Can you work these out from the model? Positions are in its coordinate system, mm. A direction names the side the tool comes from. Round coordinates to 2 decimals unless told otherwise and drop trailing zeros. Write each loop counter-clockwise with the first axis right and the second up, starting at its lowest first coordinate (ties: lowest second). Pieces come first, ordered by that corner, then holes. Notation, with made-up numbers: M 73,32 L 90,32 A13 ccw 90,51 Z; hole C 29,-15.5 d1. An arc over 180 degrees is marked long. Answer in a Markdown table with one row per item. Add a question column.
(1) Suppose I cut it at B-B, the plane z = 16. Write out the boundary of the cut face in (x, y), then the cut area to 3 significant figures.
(2) For faces 5 (the face through (24.653, 28.694, 7.972)), 6 (the face through (28, 2, 0)), 7 (the face through (28, 17, 18)), 8 (the face through (-13, 36, 8)), which set-ups out of +Z, -Z, +X, -X, +Y, -Y let a thin tool reach every point of the face, with its end or its side?
(3) If we mould it in two halves opening along Y, with no side actions, what happens to faces 1 (the face through (32.77, 18.5, -13.25)), 2 (the face through (-27.4, 35.43, -7.97)), 3 (the face through (2.176, 36.842, -7.972)), 4 (the face through (21, 39, 8))? For each: released by +Y, released by -Y, zero draft, split by the parting line, or undercut.
(4) Suppose I cut it at C-C, the plane x = -7.5. Write out the boundary of the cut face in (y, z), then the cut area to 3 significant figures.
(5) Suppose I cut it at D-D, the plane z = 25. Write out the boundary of the cut face in (x, y), then the cut area to 3 significant figures.
(6) If I drill on probe 1 along Z at (x, y) = (11, 3.1); probe 2 along Z at (x, y) = (24, 18); probe 3 along Z at (x, y) = (9.5, 48), over which ranges is the centre line in solid material (lowest first)?
(7) Suppose I cut it at A-A, the plane y = 17. Write out the boundary of the cut face in (x, z), then the cut area to 3 significant figures.
(8) I'm going to push flat-ended pins straight in: pin 1 (14 mm diameter, centred on x = 12.5, y = 19.5, fed in from -Z); pin 2 (6 mm diameter, centred on x = 22, z = -18.5, fed in from -Y); pin 3 (6 mm diameter, centred on x = 4.5, z = 2, fed in from +Y); pin 4 (1.2 mm diameter, centred on y = 2.5, z = 5.5, fed in from +X). Where does each tip first touch, or does it pass through?
from build123d import *

# Parameters (mm, degrees)
SKETCH1_R           = 3.5
BOSS_EXTRUDE1_DEPTH = 4
BOSS_EXTRUDE2_DEPTH = 4
SKETCH6_R           = 5
BOSS_EXTRUDE3_DEPTH = 12


with BuildPart() as part:
    # Sketch1 → Boss-Extrude1 (new body)
    with BuildSketch(Plane(origin=(0, 0, 0), x_dir=(1, 0, 0), z_dir=(0, 1, 0))):
        Polygon((-28, 23), (-18, 33), (12, 33), (28, 17), (28, -17), (12, -33), (-18, -33), (-28, -23), align=None)
        with Locations((11, 25)):
            Circle(SKETCH1_R, mode=Mode.SUBTRACT)
        with Locations((11, -25)):
            Circle(SKETCH1_R, mode=Mode.SUBTRACT)
        with Locations((-16, -25)):
            Circle(SKETCH1_R, mode=Mode.SUBTRACT)
        with Locations((-16, 25)):
            Circle(SKETCH1_R, mode=Mode.SUBTRACT)
    extrude(amount=BOSS_EXTRUDE1_DEPTH)

    # Sketch2 → Boss-Extrude2 (add)
    with BuildSketch(Plane.XY.offset(6)):
        with BuildLine():
            Line((-28, 34), (-28, 4))
            Line((-28, 4), (28, 4))
            Line((28, 4), (32.615384615, 15.076923077))
            ThreePointArc((32.615384615, 15.076923077), (23.839748528, 14.226499019), (28, 22))
            Line((28, 22), (21.211145618, 35.577708764))
            ThreePointArc((21.211145618, 35.577708764), (21.053502021, 36.012630114), (21, 36.472135955))
            Line((21, 36.472135955), (21, 41.5))
            ThreePointArc((21, 41.5), (10.03689158, 50.886656154), (2.450670789, 38.608695652))
            ThreePointArc((2.450670789, 38.608695652), (2.160694556, 36.820464351), (0.54554885, 36))
            Line((0.54554885, 36), (-26, 36))
            ThreePointArc((-26, 36), (-27.414213562, 35.414213562), (-28, 34))
        make_face()
    boss_extrude2 = extrude(amount=BOSS_EXTRUDE2_DEPTH)

    # Sketch6 → Boss-Extrude3 (add)
    with BuildSketch(Plane.XY.offset(6)):
        with Locations((28, 17)):
            Circle(SKETCH6_R)
    boss_extrude3 = extrude(amount=BOSS_EXTRUDE3_DEPTH)

    # Mirror1: Boss-Extrude2 across plane
    add(boss_extrude2.mirror(Plane.XY))

    # Mirror2: Boss-Extrude3 across plane
    add(boss_extrude3.mirror(Plane.XY))


solid = part.part
Calculated:
| question | item | result |
|---|---|---|
| 1 | outline | M -28,0 L 28,0 L 28,4 L -28,4 Z; C 28,17 d10 |
| 1 | area | 303 mm² |
| 2 | face 5 | +Z, -Z, +X, +Y |
| 2 | face 6 | +Z, -Z, +X, -Y |
| 2 | face 7 | +Z, +X, -X, +Y |
| 2 | face 8 | +Z, -Z, -X, +Y |
| 3 | face 1 | undercut |
| 3 | face 2 | released by +Y |
| 3 | face 3 | undercut |
| 3 | face 4 | zero draft |
| 4 | outline | M 0,-33 L 4,-33 L 4,-10 L 36,-10 L 36,-6 L 4,-6 L 4,6 L 36,6 L 36,10 L 4,10 L 4,33 L 0,33 Z |
| 4 | area | 520 mm² |
| 5 | outline | M -26,0 L -19.5,0 L -19.5,4 L -26,4 Z; M -12.5,0 L 7.5,0 L 7.5,4 L -12.5,4 Z; M 14.5,0 L 20,0 L 20,4 L 14.5,4 Z |
| 5 | area | 128 mm² |
| 6 | probe 1 | -33 to -28.5, -21.5 to 21.5, 28.5 to 33 |
| 6 | probe 2 | -18 to -6, 6 to 18 |
| 6 | probe 3 | -10 to -6, 6 to 10 |
| 7 | outline | M -28,-10 L 23,-10 L 23,-18 L 33,-18 L 33,-6 L -28,-6 Z; M -28,6 L 33,6 L 33,18 L 23,18 L 23,10 L -28,10 Z |
| 7 | area | 648 mm² |
| 8 | pin 1 | z = -10 |
| 8 | pin 2 | y = 0 |
| 8 | pin 3 | y = 4 |
| 8 | pin 4 | x = 28 |
